from build123d import *

# Parameters (mm, degrees)
SKETCH_1_W      = 15
SKETCH_1_H      = 15
EXTRUDE_1_DEPTH = 310
EXTRUDE_3_DEPTH = 17
EXTRUDE_4_DEPTH = 17


with BuildPart() as part:
    # 草图1 → 凸台-拉伸1 (new body)
    with BuildSketch(Plane(origin=(0, 0, 0), x_dir=(1, 0, 0), z_dir=(0, 1, 0))):
        with Locations((7.5, 7.5)):
            Rectangle(SKETCH_1_W, SKETCH_1_H)
    extrude(amount=EXTRUDE_1_DEPTH)

    # 草图3 → 凸台-拉伸3 (add)
    with BuildSketch(Plane(origin=(0, 80, 0), x_dir=(-1, 0, 0), z_dir=(0, -1, 0))):
        Polygon((-7.5, 31.54163056), (-31.54163056, 7.5), (-7.5, -16.54163056), (16.54163056, 7.5), align=None)
    extrude(amount=-EXTRUDE_3_DEPTH)

    # 草图4 → 凸台-拉伸4 (add)
    with BuildSketch(Plane(origin=(0, 230, 0), x_dir=(1, 0, 0), z_dir=(0, 1, 0))):
        Polygon((7.5, 31.54163056), (-16.54163056, 7.5), (7.5, -16.54163056), (31.54163056, 7.5), align=None)
    extrude(amount=-EXTRUDE_4_DEPTH)


solid = part.part
Design review of the part built by this model. Coordinates are the model's own, in mm. A direction names the side the tool comes from. Give positions to 0.01 mm unless a question says otherwise; leave off trailing zeros. Order: outer loops, then holes, each group sorted by start corner. A loop starts at its lowest first (then second) coordinate and runs counter-clockwise, first axis right, second up. Notation, with made-up numbers: (23.25, -20) - (52.25, -20) arc R20 cw to (52.25, 11) - close; hole circle Ø2 at (70, 84). An arc over 180 degrees is marked (long way). Use CSV: the item, a comma, the result in double quotes. Start each with the question number.
Q1. Take a section at B-B (x = 21). State the section outline as (y, z) points, and give its area (3 significant figures).
Q2. For line 1 (Y direction, x = 8, z = 1); line 2 (Z direction, x = 7, y = 33); line 3 (X direction, y = 98.5, z = -1), list the stretches that pass through material, from the lowest coordinate up.
Q3. Take a section at A-A (z = -26). State the section outline as (x, y) points.
Q4. Take a section at C-C (z = -12). State the section outline as (x, y) points, and give its area (3 significant figures).
Q5. For P1, Ø16.5, axis at y = 262.5, z = -10, coming from the -X side; P2, Ø6, axis at x = 1, z = -21, coming from the -Y side; P3, Ø12, axis at x = 10, y = 161.5, coming from the +Z side; P4, Ø24, axis at x = 15.5, z = -10.5, coming from the -Y side, all flat-tipped, find the tip position at first contact; note any pin that passes through.
Q6. Machinability: for faces 4 (the face through (15, 154, -7)), 5 (the face through (-4, 213, -8)), 6 (the face through (15, 39, -7)), 7 (the face through (7, 269, -15)), which of the approach directions +Z, -Z, +X, -X, +Y, -Y give a long, thin tool a straight path to every point of the face, cutting with its end or side? Answer none if there is none.
Q7. Draft analysis for pull direction Y (two halves, no side actions). For faces 1 (the face through (7, 0, -8)), 2 (the face through (-4.35, 88.38, 4.69)), 3 (the face through (0, 154, -7)), state which applies: pulls with the +Y half, pulls with the -Y half, needs draft (parallel to the pull), parting line crosses it, or undercut.
Q8. Take a section at D-D (y = 145). State the section outline as (x, z) points.
Calculated:
1,outline,"(80, -18.04) - (97, -18.04) - (97, 3.04) - (80, 3.04) - close; (213, -18.04) - (230, -18.04) - (230, 3.04) - (213, 3.04) - close"
1,area,"717 mm²"
2,line 1,"y = 80 to 97, 213 to 230"
2,line 2,"z = -15 to 0"
2,line 3,"x = 0 to 15"
3,outline,"(1.96, 80) - (13.04, 80) - (13.04, 97) - (1.96, 97) - close; (1.96, 213) - (13.04, 213) - (13.04, 230) - (1.96, 230) - close"
4,outline,"(-12.04, 80) - (0, 80) - (0, 0) - (15, 0) - (15, 80) - (27.04, 80) - (27.04, 97) - (15, 97) - (15, 213) - (27.04, 213) - (27.04, 230) - (15, 230) - (15, 310) - (0, 310) - (0, 230) - (-12.04, 230) - (-12.04, 213) - (0, 213) - (0, 97) - (-12.04, 97) - close"
4,area,"5,470 mm²"
5,P1,"stops at x = 0"
5,P2,"stops at y = 80"
5,P3,"stops at z = 0"
5,P4,"stops at y = 0"
6,face 4,"+Z, -Z, +X"
6,face 5,"none"
6,face 6,"+Z, -Z, +X, -Y"
6,face 7,"-Z, +X, -X, +Y"
7,face 1,"pulls with the -Y half"
7,face 2,"needs draft"
7,face 3,"undercut"
8,outline,"(0, -15) - (15, -15) - (15, 0) - (0, 0) - close"
